```python
from build123d import *

# Parameters (mm, degrees)
SKETCH_1_R               = 28.5
EXTRUDE_1_DEPTH          = 45
EXTRUDE_2_DEPTH          = 1
EXTRUDE_2_DEPTH_BACK     = 30
SKETCH_2_R               = 17.5
PATTERN_CIRCULAR_2_COUNT = 6
SKETCH_11_2_R            = 1.5
CUT_EXTRUDE_1_DEPTH      = 5
PATTERN_CIRCULAR_3_COUNT = 6
SKETCH_13_2_R            = 2
CUT_EXTRUDE_2_DEPTH      = 4
PATTERN_CIRCULAR_4_COUNT = 4
CUT_EXTRUDE_START        = -1
SKETCH_18_W              = 15
SKETCH_18_H              = 10
CUT_EXTRUDE_3_DEPTH      = 6


with BuildPart() as part:
    # Sketch 1 → Extrude 1 (new body)
    with BuildSketch(Plane(origin=(0, 0, 0), x_dir=(1, 0, 0), z_dir=(0, 1, 0))):
        with Locations(Location((0, 0, 0), (0, 0, 90))):
            Circle(SKETCH_1_R)
    extrude(amount=EXTRUDE_1_DEPTH)

    # Sketch 2 → Extrude 2 (add, two sides: drawn at the far end of the back side and taken through both)
    with BuildSketch(Plane(origin=(0, 45, 0), x_dir=(1, 0, 0), z_dir=(0, 1, 0)).offset(-EXTRUDE_2_DEPTH_BACK)):
        with Locations(Location((0, 0, 0), (0, 0, 270))):
            Circle(SKETCH_2_R)
    extrude(amount=EXTRUDE_2_DEPTH + EXTRUDE_2_DEPTH_BACK)

    # Sketch 12 → Hole Wizard M3 _2 (revolve, cut)
    with BuildSketch(Plane(origin=(0, 45, -25), x_dir=(0, 0, 1), z_dir=(1, 0, 0))):
        Polygon((0, 0), (0, 5.751075774), (1.25, 5), (1.25, 0.275), (1.525, 0), align=None)
    hole_wizard_m3_2 = revolve(axis=Axis((0, 51.35, -25), (0, -1, 0)), mode=Mode.SUBTRACT)

    # Pattern Circular 2: Hole Wizard M3 _2 ×6 about axis
    pattern_circular_2_axis = Axis((0, 0, 0), (0, 1, 0))
    for i in range(1, PATTERN_CIRCULAR_2_COUNT):
        add(hole_wizard_m3_2.rotate(pattern_circular_2_axis, i * 360 / PATTERN_CIRCULAR_2_COUNT), mode=Mode.SUBTRACT)

    # Sketch 11_2 → Cut-Extrude 1 (cut)
    with BuildSketch(Plane(origin=(0, 45, 0), x_dir=(1, 0, 0), z_dir=(0, 1, 0))):
        with Locations(Location((6.470476128, 24.148145657, 0), (0, 0, 270))):
            Circle(SKETCH_11_2_R)
        with Locations(Location((-6.470476128, -24.148145657, 0), (0, 0, 270))):
            Circle(SKETCH_11_2_R)
    extrude(amount=-CUT_EXTRUDE_1_DEPTH, mode=Mode.SUBTRACT)

    # Sketch 14 → Hole Wizard M3 _3 (revolve, cut)
    with BuildSketch(Plane(origin=(-13.5, 46, 0), x_dir=(0, 0, 1), z_dir=(1, 0, 0))):
        Polygon((0, 0), (0, 5.751075774), (1.25, 5), (1.25, 0.275), (1.525, 0), align=None)
    hole_wizard_m3_3 = revolve(axis=Axis((-13.5, 52.35, 0), (0, -1, 0)), mode=Mode.SUBTRACT)

    # Pattern Circular 3: Hole Wizard M3 _3 ×6 about axis
    pattern_circular_3_axis = Axis((0, 0, 0), (0, 1, 0))
    for i in range(1, PATTERN_CIRCULAR_3_COUNT):
        add(hole_wizard_m3_3.rotate(pattern_circular_3_axis, i * 360 / PATTERN_CIRCULAR_3_COUNT), mode=Mode.SUBTRACT)

    # Sketch 13_2 → Cut-Extrude 2 (cut)
    with BuildSketch(Plane(origin=(0, 46, 0), x_dir=(1, 0, 0), z_dir=(0, 1, 0))):
        with Locations(Location((0, -12.15, 0), (0, 0, 270))):
            Circle(SKETCH_13_2_R)
        with Locations(Location((-10.522208656, 6.075, 0), (0, 0, 270))):
            Circle(SKETCH_13_2_R)
        with Locations(Location((10.522208656, 6.075, 0), (0, 0, 270))):
            Circle(SKETCH_13_2_R)
    extrude(amount=-CUT_EXTRUDE_2_DEPTH, mode=Mode.SUBTRACT)

    # Sketch 17 → Hole Wizard M3 _4 (revolve, cut)
    with BuildSketch(Plane(origin=(13.435028843, 0, 13.435028843), x_dir=(0, 0, -1), z_dir=(1, 0, 0))):
        Polygon((0, 0), (0, 4.751075774), (1.25, 4), (1.25, 0.275), (1.525, 0), align=None)
    hole_wizard_m3_4 = revolve(axis=Axis((13.435028843, -6.35, 13.435028843), (0, 1, 0)), mode=Mode.SUBTRACT)

    # Pattern Circular 4: Hole Wizard M3 _4 ×4 about axis
    pattern_circular_4_axis = Axis((0, 0, 0), (0, 1, 0))
    for i in range(1, PATTERN_CIRCULAR_4_COUNT):
        add(hole_wizard_m3_4.rotate(pattern_circular_4_axis, i * 360 / PATTERN_CIRCULAR_4_COUNT), mode=Mode.SUBTRACT)

    # Sketch 18 → Cut-Extrude 3 (cut)
    with BuildSketch(Plane.XZ.offset(CUT_EXTRUDE_START)):
        with Locations((0, -23.5)):
            Rectangle(SKETCH_18_W, SKETCH_18_H)
        Polygon((11.748383566, 27.027309958), (10.227092755, 17.143703619), (-4.598316754, 19.425639836), (-3.077025943, 29.309246175), align=None)
    extrude(amount=-CUT_EXTRUDE_3_DEPTH, mode=Mode.SUBTRACT)


solid = part.part
```
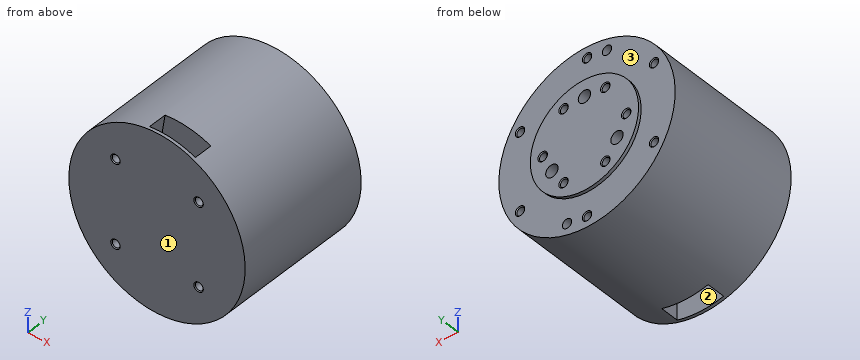
Input: part model. Units: mm. Frame: model coordinates. Face numbers are marked on the shaded views. Give positions to 0.01 mm unless a question says otherwise; leave off trailing zeros. Order: outer loops, then holes, each group sorted by start corner. A loop starts at its lowest first (then second) coordinate and runs counter-clockwise, first axis right, second up.
1. Cut plane B-B (y = 10). Return loops of the section in (x, z).
Computed:
outline: circle Ø57 at (0, 0)
2. Pin query (flat end, axial travel): pin 1 Ø1 at (y, z) = (15.5, 10.5) entering from +X; pin 2 Ø2 at (x, z) = (13.44, 13.44) entering from -Y; pin 3 Ø5 at (y, z) = (4.5, -21.5) entering from -X. Return the tip coordinate at first contact, or that it passes through.
Computed:
pin 1: stops at x = 26.69
pin 2: stops at y = 4.15
pin 3: stops at x = -21.24
3. Cut plane A-A (z = 8). Return loops of the section in (x, y).
Computed:
outline: (-27.35, 0) - (27.35, 0) - (27.35, 45) - (15.56, 45) - (15.56, 46) - (-15.56, 46) - (-15.56, 45) - (-27.35, 45) - close
4. Draft query along Y for the marked faces 1, 2 and 3. Return one class per face: released by +Y, released by -Y, zero draft, split by the parting line, or undercut.
Computed:
face 1: released by -Y
face 2: undercut
face 3: released by +Y
5. Line query: probe 1 along Z at (x, y) = (-6, 42); probe 2 along Y at (x, z) = (-5, -23.5); probe 3 along Z at (x, y) = (1, 44). Output: solid intervals per line, ascending.
Computed:
probe 1: z = -27.86 to -12.69, -10.69 to 10.69, 12.69 to 22.72, 25.57 to 27.86
probe 2: y = 0 to 1, 7 to 45
probe 3: z = -28.48 to -25.75, -24.25 to 10.42, 13.88 to 24.25, 25.75 to 28.48
